For this review, take the finished solid that the model builds, in its own axes (mm). A direction names the side the tool comes from. Round coordinates to 2 decimals unless told otherwise and drop trailing zeros. Order: outer loops, then holes, each group sorted by start corner. A loop starts at its lowest first (then second) coordinate and runs counter-clockwise, first axis right, second up. Notation, with made-up numbers: M 81,33.5 L 110,33.5 A15 ccw 110,57.5 Z; hole C 53,-0.5 d4. An arc over 180 degrees is marked long. Use a Markdown table: item, result.
from build123d import *

# Parameters (mm, degrees)
SKETCH003_R     = 1.5
PAD002_DEPTH    = 6
SKETCH004_W     = 7
SKETCH004_H     = 2.5
POCKET001_DEPTH = 1
SKETCH005_W     = 7
SKETCH005_H     = 1.62
PAD003_DEPTH    = 0.4


with BuildPart() as part:
    # Sketch003 → Pad002 (new body)
    with BuildSketch(Plane.XY):
        with BuildLine():
            Line((-12, 3.8), (12, 3.8))
            Line((12, 3.8), (12, 9))
            ThreePointArc((12, 9), (11.12132, 11.12132), (9, 12))
            Line((9, 12), (-9, 12))
            ThreePointArc((-9, 12), (-11.12132, 11.12132), (-12, 9))
            Line((-12, 9), (-12, 3.8))
        make_face()
        with Locations((-8, 6.5)):
            Circle(SKETCH003_R, mode=Mode.SUBTRACT)
        with Locations((8, 6.5)):
            Circle(SKETCH003_R, mode=Mode.SUBTRACT)
    extrude(amount=PAD002_DEPTH)

    # Sketch004 (on Face1 of Pad002) → Pocket001 (cut)
    with BuildSketch(Plane.XZ.offset(-3.8)):
        with Locations((0, 3.25)):
            Rectangle(SKETCH004_W, SKETCH004_H)
    extrude(amount=-POCKET001_DEPTH, mode=Mode.SUBTRACT)

    # Sketch005 (on Face1 of Pocket001) → Pad003 (join)
    with BuildSketch(Plane.XZ.offset(-3.8)):
        with Locations((1, 3.25)):
            Rectangle(SKETCH005_W, SKETCH005_H)
    extrude(amount=PAD003_DEPTH)


solid = part.part
Q1. Wall thickness on line 1 along Y through (x, z) = (-8, 1.4); line 2 along Z through (x, y) = (-1.5, 4); line 3 along Y through (x, z) = (5.25, 0.85): over which ranges is each line inside the solid? List them lowest first. Write a range as [from, to].
Determined:
| item | result |
|---|---|
| line 1 | y = [3.8, 5], [8, 12] |
| line 2 | z = [0, 2], [4.5, 6] |
| line 3 | y = [3.8, 12] |
Q2. Add section B-B (y = 4.25). Write out the cut boundary in (x, z).
Determined:
| item | result |
|---|---|
| outline | M -12,0 L 12,0 L 12,6 L -12,6 Z; hole M -3.5,2 L 3.5,2 L 3.5,4.5 L -3.5,4.5 Z |
Q3. Add section D-D (y = 7.5). Write out the cut boundary in (x, z), then the cut area to 3 significant figures.
Determined:
| item | result |
|---|---|
| outline | M -12,0 L -9.12,0 L -9.12,6 L -12,6 Z; M -6.88,0 L 6.88,0 L 6.88,6 L -6.88,6 Z; M 9.12,0 L 12,0 L 12,6 L 9.12,6 Z |
| area | 117 mm^2 |
Q4. Add section C-C (z = 1.25). Write out the cut boundary in (x, y).
Determined:
| item | result |
|---|---|
| outline | M -12,3.8 L 12,3.8 L 12,9 A3 ccw 9,12 L -9,12 A3 ccw -12,9 Z; hole C -8,6.5 d3; hole C 8,6.5 d3 |
Q5. Add section A-A (x = -8). Write out the cut boundary in (y, z).
Determined:
| item | result |
|---|---|
| outline | M 3.8,0 L 5,0 L 5,6 L 3.8,6 Z; M 8,0 L 12,0 L 12,6 L 8,6 Z |
Q6. Draft analysis for pull direction Z (two halves, no side actions). For faces 4 (the flat face through (-12, 6, 3)), 5 (the flat face through (0, 8, 6)), 6 (the flat face through (0, 8, 0)), 7 (the flat face through (0, 4, 4.5)), state which applies: pulls with the +Z half, pulls with the -Z half, needs draft (parallel to the pull), parting line crosses it, or undercut.
Determined:
| item | result |
|---|---|
| face 4 | needs draft |
| face 5 | pulls with the +Z half |
| face 6 | pulls with the -Z half |
| face 7 | undercut |
Q7. Clearance check with flat-ended pins moving along their axes: pin 1 (1 mm diameter, centred on y = 10.5, z = 5, fed in from +X); pin 2 (2.5 mm diameter, centred on x = -8, y = 6.5, fed in from +Z). State where each tip first meets the part, or that it passes through.
Determined:
| item | result |
|---|---|
| pin 1 | stops at x = 11.83 |
| pin 2 | passes through |
Q8. Machinability: for faces 1 (the cylindrical face through (-11.1, 11.14, 2.96)), 2 (the flat face through (-3.5, 4, 3)), 3 (the flat face through (3.5, 4, 3)), which of the approach directions +Z, -Z, +X, -X, +Y, -Y give a long, thin tool a straight path to every point of the face, cutting with its end or side? Answer none if there is none.
Determined:
| item | result |
|---|---|
| face 1 | +Z, -Z, -X, +Y |
| face 2 | -Y |
| face 3 | none |
